Autodesk Inventor part; units mm, degrees
ref_plane "Work Plane1" through (0, 0, 10) normal (0, 0, 1) x (1, 0, 0)
ref_plane "YZ Plane" through (0, 0, 0) normal (1, 0, 0) x (0, 1, 0)
ref_plane "XZ Plane" through (0, 0, 0) normal (0, 1, 0) x (-1, 0, 0)
sketch "Sketch1" plane through (0, 0, 0) normal (0, 0, 1) x (1, 0, 0)
  line L0 (0, 0) -> (17.5, 0)
  line L1 (17.5, 0) -> (17.5, 8)
  line L2 (17.5, 8) -> (0, 8)
  line L3 (0, 8) -> (0, 0)
  line L4 (0, 8) -> (16.5, 8)
  line L5 (16.5, 8) -> (16.5, 3)
  line L6 (16.5, 3) -> (0, 3)
  line L7 (0, 3) -> (0, 8)
  line L8 (0, 3) -> (7.5, 3)
  line L9 (7.5, 3) -> (7.5, 5)
  line L10 (7.5, 5) -> (0, 5)
  line L11 (0, 5) -> (0, 3)
  line L12 (7.5, 5) -> (5.5, 8)
  line L13 (0, 8) -> (2.5, 8)
  line L14 (2.5, 8) -> (2.5, 0)
  line L15 (2.5, 0) -> (0, 0)
  line L16 (0, 0) -> (0, 8)
  point P0 (16.5, 5.5)
  dimension "d0" = 17.5
  dimension "d1" = 8
  dimension "d2" = 1
  dimension "d3" = 3
  dimension "d4" = 7.5
  dimension "d5" = 2
  dimension "d6" = 5.5
  dimension "d7" = 2.5
revolve "Revolution1" add sketch "Sketch1" angle 360 about axis through (0, 8, 0) along (0, -1, 0) contours L14 L6 L5 L2 L1 L0 | L14 L10 L9 L6 | L14 L2 L12 L10
chamfer "Chamfer1" distance 2 angle 45 1 edges at (-17.5, 0, 0)
fillet "Fillet1" radius 1 1 edges at (-16.5, 3, 0)
sketch "Sketch2" plane through (0, 0, 0) normal (0, -1, 0) x (1, 0, 0)
  circle A0 centre (0, 0) radius 12.5 construction
  line L0 (0, 12.5) -> (0, 0) construction
  circle A1 centre (0, 0) radius 2.5
  circle A2 centre (0, 0) radius 15.5
  circle A3 centre (0, 0) radius 15.5
  line L1 (0, 0) -> (-8.8388, 8.8388) construction
  circle A4 centre (-8.8388, 8.8388) radius 1.5
  circle A5 centre (-8.8388, -8.8388) radius 1.5
  circle A6 centre (8.8388, -8.8388) radius 1.5
  circle A7 centre (8.8388, 8.8388) radius 1.5
  line L2 (-8.4184, 13.0146) -> (-13.0146, 8.4184) construction
  line L3 (8.4184, 13.0146) -> (13.0146, 8.4184) construction
  circle A8 centre (0, 0) radius 9.5 construction
  circle A9 centre (0, 21.433) radius 11.933
  circle A10 centre (-21.433, 0) radius 11.933
  circle A11 centre (0, -21.433) radius 11.933
  circle A12 centre (21.433, 0) radius 11.933
  circle A13 centre (0, 0) radius 5.5
  point P0 (-10.7165, 10.7165)
  point P1 (-8.4421, -12.9993)
  point P2 (8.4421, -12.9993)
  dimension "d13" = 25
  dimension "d15" = 45
  dimension "d16" = 3
  dimension "d19" = 360
  dimension "d21" = 6.5
  dimension "d22" = 19
  dimension "d25" = 360
  dimension "d27" = 11
extrude "Extrusion1" cut sketch "Sketch2" against normal blind 7 contours A1 | A2 A12 | A2 A12 | A11 A2 | A2 A11 | A10 A2 | A2 A10 | A4 | A5 | A6 | A7 | A13
extrude "Extrusion2" cut sketch "Sketch2" against normal blind 0.5 contours A9 A2 | A2 A9
ref_plane "Work Plane1" through (0, 0, 10) normal (0, 0, 1) x (1, 0, 0)
sketch "Sketch3" plane through (0, 0, 10) normal (0, 0, 1) x (1, 0, 0)
  line L0 (-17.5, 8) -> (17.5, 8)
  line L1 (0, 8) -> (0, 0) construction
  line L2 (-4.25, 5.25) -> (4.25, 5.25) construction
  line L3 (5.5, 0) -> (-5.5, 0)
  line L4 (-4.25, 3) -> (4.25, 3)
  line L5 (4.25, 7.5) -> (-4.25, 7.5)
  arc A0 (-4.25, 7.5) -> (-4.25, 3) centre (-4.25, 5.25) ccw
  arc A1 (4.25, 3) -> (4.25, 7.5) centre (4.25, 5.25) ccw
  line L6 (8.7938, 0.5) -> (-8.7938, 0.5)
  point P0 (0, 5.25)
  dimension "d33" = 2.5
  dimension "d34" = 2.25
  dimension "d35" = 8.5
extrude "Extrusion3" cut sketch "Sketch3" along normal through all
properties part number "Base" material "Stainless Steel"
Read the model definition and answer for the solid it produces. Units are mm, in the model's axes. A direction names the side the tool comes from. Round coordinates to 2 decimals unless told otherwise and drop trailing zeros. Write each loop counter-clockwise with the first axis right and the second up, starting at its lowest first coordinate (ties: lowest second). Pieces come first, ordered by that corner, then holes. Notation, with made-up numbers: (9, 75.5) - (37, 75.5) arc R16 cw to (37, 85.5) - close; hole circle Ø2 at (44.25, 85). An arc over 180 degrees is marked (long way). One line per item, written item: value.
Q1. Find section B-B (z = -0.5). Count the separate pieces of the cut face and the enclosed holes in it, and give its area (3 significant figures).
The answers:
separate pieces: 4
enclosed holes: 0
area: 46.3 mm2
Q2. For a pull along X with two mould halves and no side action, classify faces 1 (the flat face through (-17, 7, 0)), 2 (the conical face through (-0.2, 0.8, 16.3)), 3 (the cylindrical face through (0.2, 1.9, -9.5)) as pulls with the +X half, pulls with the -X half, needs draft (parallel to the pull), parting line crosses it, or undercut.
The answers:
face 1: needs draft
face 2: parting line crosses it
face 3: undercut
Q3. Each of these flat-tipped pins is pushed along its axis until it touches: P1, Ø1, axis at x = -10.5, z = -11.5, coming from the +Y side; P2, Ø1.1, axis at x = -15, z = 2.5, coming from the -Y side (3 decimals); P3, Ø3.5, axis at x = 0, z = -1.5, coming from the -Y side; P4, Ø0.5, axis at x = -0.5, z = 17, coming from the -Y side. Where does it stop, or does it pass through?
The answers:
P1: stops at y = 3.18
P2: passes through
P3: stops at y = 7
P4: stops at y = 1.26
Q4. Find section A-A (y = 1.25). Determine the outline of the cut face in (x, z).
The answers:
outline: (-13.94, -9.29) arc R16.75 ccw to (-9.29, -13.94) arc R11.93 cw to (9.29, -13.94) arc R16.75 ccw to (13.94, -9.29) arc R11.93 cw to (13.94, 9.29) arc R16.75 ccw to (-13.94, 9.29) arc R11.93 cw to start; hole circle Ø3 at (-8.84, -8.84); hole circle Ø3 at (-8.84, 8.84); hole circle Ø11 at (0, 0); hole circle Ø3 at (8.84, -8.84); hole circle Ø3 at (8.84, 8.84)
Q5. Straight lines are drawn through the part: line 1 (Z direction, x = 0, y = 3.5); line 2 (Y direction, x = 1, z = 13); line 3 (Y direction, x = -9, z = -4). For each, find the intervals that lie inside material, in ascending order. Write a range as from..to.
The answers:
line 1: z = -7.5..-5.5, 5.5..7.5
line 2: y = 0.5..3
line 3: y = 0..3
Q6. Which of the six approach directions +Z, -Z, +X, -X, +Y, -Y give full straight-line access (tool end or side, diameter ignored) to faces 4 (the cylindrical face through (6.5, 5.3, 15.9)), 5 (the flat face through (-3, 7, 0)), 6 (the cylindrical face through (-7.493, 4.014, -0.33))?
The answers:
face 4: +Z
face 5: -Y
face 6: +Y
